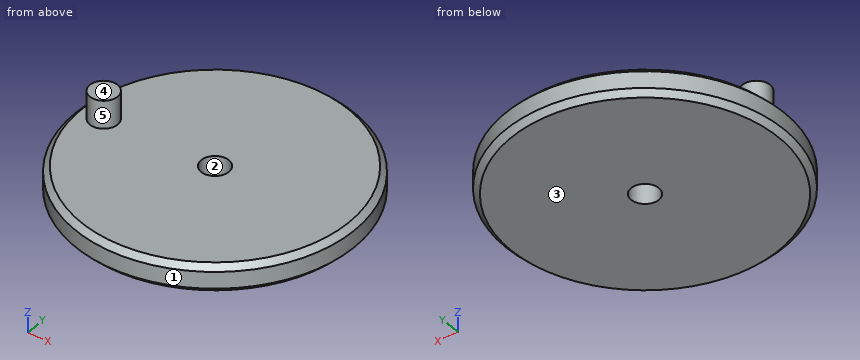
```python
from build123d import *

# Parameters (mm, degrees)
SKETCH1_R           = 25
SKETCH1_R_2         = 2.5
BOSS_EXTRUDE1_DEPTH = 5
SKETCH2_R           = 2.5
BOSS_EXTRUDE2_DEPTH = 5
CHAMFER1_SIZE       = 1


with BuildPart() as part:
    # Sketch1 → Boss-Extrude1 (new body)
    with BuildSketch(Plane.XY):
        Circle(SKETCH1_R)
        Circle(SKETCH1_R_2, mode=Mode.SUBTRACT)
    extrude(amount=BOSS_EXTRUDE1_DEPTH)

    # Sketch2 → Boss-Extrude2 (add)
    with BuildSketch(Plane.XY.offset(5)):
        with Locations((-20, 0)):
            Circle(SKETCH2_R)
    extrude(amount=BOSS_EXTRUDE2_DEPTH)

    # Chamfer1
    chamfer1_edges = [part.edges().sort_by_distance(p)[0] for p in [
        (-25, 0, 0),
        (-25, 0, 5),
    ]]
    chamfer(chamfer1_edges, length=CHAMFER1_SIZE)


solid = part.part
```
For this review, take the finished solid that the model builds, in its own axes (mm). Face numbers are marked on the shaded views. A direction names the side the tool comes from. Coordinates: 2 decimals unless noted, no trailing zeros. Write each loop counter-clockwise with the first axis right and the second up, starting at its lowest first coordinate (ties: lowest second). Pieces come first, ordered by that corner, then holes.
(1) Add section C-C on z = 8.25. Give the boundary of the cut face in (x, y), then the cut area to 3 significant figures.
(2) For pin 1 Ø1 at (x, y) = (14.5, -8.5) entering from +Z; pin 2 Ø6 at (y, z) = (-8.5, 4) entering from +X; pin 3 Ø2 at (x, z) = (14, 1.5) entering from -Y, all flat-tipped, find the tip position at first contact; note any pin that passes through.
(3) Add section A-A on x = 0. Give the boundary of the cut face in (y, z), then the cut area to 3 significant figures.
(4) Wall thickness on probe 1 along Y at (x, z) = (0, 1.4); probe 2 along Z at (x, y) = (-3.5, 3); probe 3 along X at (y, z) = (-4, 4.25): over which ranges is each line inside the solid? List them lowest first.
(5) Add section B-B on y = 0. Give the boundary of the cut face in (x, z), then the cut area to 3 significant figures.
(6) Tool access review of the marked faces 4 and 5: name each direction out of +Z, -Z, +X, -X, +Y, -Y from which nothing blocks a thin tool from reaching the whole face with its end or side.
(7) The part is to be moulded in two halves that separate along X. For the marked faces 1, 2 and 3, say which applies: +X half, -X half, draft (parallel to the pull), parting line (faces both ways), or undercut.
Answer sheet:
1. outline: circle Ø5 at (-20, 0)
1. area: 19.6 mm2
2. pin 1: stops at z = 5
2. pin 2: stops at x = 24.39
2. pin 3: stops at y = -21.35
3. outline: (-25, 1) - (-24, 0) - (-2.5, 0) - (-2.5, 5) - (-24, 5) - (-25, 4) - close; (2.5, 0) - (24, 0) - (25, 1) - (25, 4) - (24, 5) - (2.5, 5) - close
3. area: 223 mm2
4. probe 1: y = -25 to -2.5, 2.5 to 25
4. probe 2: z = 0 to 5
4. probe 3: x = -24.42 to 24.42
5. outline: (-25, 1) - (-24, 0) - (-2.5, 0) - (-2.5, 5) - (-17.5, 5) - (-17.5, 10) - (-22.5, 10) - (-22.5, 5) - (-24, 5) - (-25, 4) - close; (2.5, 0) - (24, 0) - (25, 1) - (25, 4) - (24, 5) - (2.5, 5) - close
5. area: 248 mm2
6. face 4: +Z, +X, -X, +Y, -Y
6. face 5: +Z
7. face 1: parting line
7. face 2: undercut
7. face 3: draft
